Check sheet for the modelled part. Datum: model origin and axes. Units: mm. Coordinates: 2 decimals unless noted, no trailing zeros. Order: outer loops, then holes, each group sorted by start corner. A loop starts at its lowest first (then second) coordinate and runs counter-clockwise, first axis right, second up.
from build123d import *

# Parameters (mm, degrees)
SKETCH1_R           = 86.25
BOSS_EXTRUDE1_DEPTH = 6
SKETCH2_R           = 1.5
CUT_EXTRUDE1_DEPTH  = 6
SKETCH3_R           = 2.25
CUT_EXTRUDE2_DEPTH  = 6
CUT_EXTRUDE3_DEPTH  = 6
FILLET1_R           = 20


with BuildPart() as part:
    # Sketch1 → Boss-Extrude1 (new body)
    with BuildSketch(Plane(origin=(0, 0, 0), x_dir=(1, 0, 0), z_dir=(0, 1, 0))):
        with BuildLine():
            Line((75.993420768, 65), (110, 65))
            Line((110, 65), (110, -65))
            Line((110, -65), (75.993420768, -65))
            ThreePointArc((75.993420768, -65), (0, -100), (-75.993420768, -65))
            Line((-75.993420768, -65), (-110, -65))
            Line((-110, -65), (-110, 65))
            Line((-110, 65), (-75.993420768, 65))
            ThreePointArc((-75.993420768, 65), (0, 100), (75.993420768, 65))
        make_face()
        Circle(SKETCH1_R, mode=Mode.SUBTRACT)
    extrude(amount=BOSS_EXTRUDE1_DEPTH)

    # Sketch2 → Cut-Extrude1 (cut)
    with BuildSketch(Plane(origin=(0, 0, 0), x_dir=(1, 0, 0), z_dir=(0, 1, 0))):
        with Locations((-95.5, 43.5)):
            Circle(SKETCH2_R)
        with Locations((95.5, 43.5)):
            Circle(SKETCH2_R)
        with Locations((95.5, -43.5)):
            Circle(SKETCH2_R)
        with Locations((-95.5, -43.5)):
            Circle(SKETCH2_R)
    extrude(amount=CUT_EXTRUDE1_DEPTH, mode=Mode.SUBTRACT)

    # Sketch3 → Cut-Extrude2 (cut)
    with BuildSketch(Plane(origin=(0, 0, 0), x_dir=(1, 0, 0), z_dir=(0, 1, 0))):
        with Locations((0, 93.125)):
            Circle(SKETCH3_R)
        with Locations((93.125, 0)):
            Circle(SKETCH3_R)
        with Locations((0, -93.125)):
            Circle(SKETCH3_R)
        with Locations((-93.125, 0)):
            Circle(SKETCH3_R)
    extrude(amount=CUT_EXTRUDE2_DEPTH, mode=Mode.SUBTRACT)

    # Sketch4 → Cut-Extrude3 (cut)
    with BuildSketch(Plane(origin=(0, 0, 0), x_dir=(1, 0, 0), z_dir=(0, 1, 0))):
        with BuildLine():
            Line((98.608905775, -36.674701114), (93.856581268, -34.510029742))
            ThreePointArc((93.856581268, -34.510029742), (100, 0), (93.856581268, 34.510029742))
            Line((93.856581268, 34.510029742), (98.608905775, 36.674701114))
            ThreePointArc((98.608905775, 36.674701114), (102.325298886, 46.608905775), (92.391094225, 50.325298886))
            Line((92.391094225, 50.325298886), (87.638769717, 48.160627513))
            ThreePointArc((87.638769717, 48.160627513), (82.248188777, 56.879130117), (75.993420768, 65))
            Line((75.993420768, 65), (110, 65))
            Line((110, 65), (110, -65))
            Line((110, -65), (75.993420768, -65))
            ThreePointArc((75.993420768, -65), (82.248188777, -56.879130117), (87.638769717, -48.160627513))
            Line((87.638769717, -48.160627513), (92.391094225, -50.325298886))
            ThreePointArc((92.391094225, -50.325298886), (102.325298886, -46.608905775), (98.608905775, -36.674701114))
        make_face()
        with BuildLine():
            Line((-98.608905775, 36.674701114), (-93.856581268, 34.510029742))
            ThreePointArc((-93.856581268, 34.510029742), (-100, 0), (-93.856581268, -34.510029742))
            Line((-93.856581268, -34.510029742), (-98.608905775, -36.674701114))
            ThreePointArc((-98.608905775, -36.674701114), (-102.325298886, -46.608905775), (-92.391094225, -50.325298886))
            Line((-92.391094225, -50.325298886), (-87.638769717, -48.160627513))
            ThreePointArc((-87.638769717, -48.160627513), (-82.248188777, -56.879130117), (-75.993420768, -65))
            Line((-75.993420768, -65), (-110, -65))
            Line((-110, -65), (-110, 65))
            Line((-110, 65), (-75.993420768, 65))
            ThreePointArc((-75.993420768, 65), (-82.248188777, 56.879130117), (-87.638769717, 48.160627513))
            Line((-87.638769717, 48.160627513), (-92.391094225, 50.325298886))
            ThreePointArc((-92.391094225, 50.325298886), (-102.325298886, 46.608905775), (-98.608905775, 36.674701114))
        make_face()
    extrude(amount=CUT_EXTRUDE3_DEPTH, mode=Mode.SUBTRACT)

    # Fillet1
    fillet1_edges = [part.edges().sort_by_distance(p)[0] for p in [
        (87.638769717, 3, -48.160627513),
        (93.856581268, 3, -34.510029742),
        (93.856581268, 3, 34.510029742),
        (87.638769717, 3, 48.160627513),
        (-87.638769717, 3, 48.160627513),
        (-93.856581268, 3, 34.510029742),
        (-93.856581268, 3, -34.510029742),
        (-87.638769717, 3, -48.160627513),
    ]]
    fillet(fillet1_edges, radius=FILLET1_R)


solid = part.part
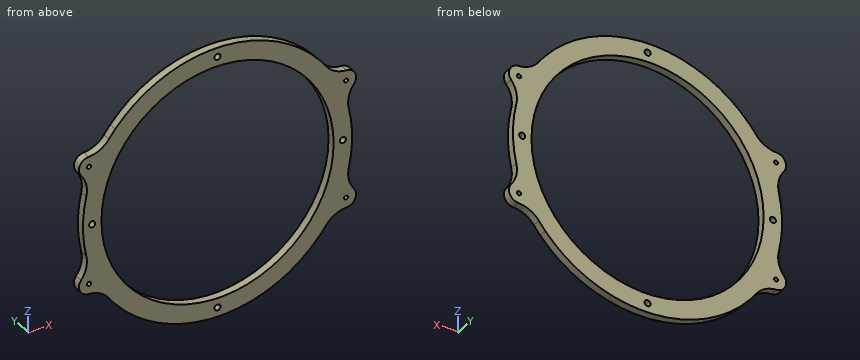
(1) Cross-section at B-B (x = -39). Enter the section's corners in (y, z).
Filled in:
outline: (0, -92.08) - (6, -92.08) - (6, -76.93) - (0, -76.93) - close; (0, 76.93) - (6, 76.93) - (6, 92.08) - (0, 92.08) - close
(2) Cross-section at C-C (y = 4). Count the separate pieces of the cut face and the enclosed holes in it, and give its area (3 significant figures).
Filled in:
separate pieces: 1
enclosed holes: 9
area: 8,830 mm2
(3) Go/stop test with flat-tipped pins: P1, Ø3, axis at y = 3.5, z = 13.5, coming from the +X side; P2, Ø1.5, axis at x = 9.5, y = 5, coming from the +Z side; P3, Ø1.5, axis at y = 0.5, z = -25.5, coming from the -X side. Record where each tip stops, or that it passes through.
Filled in:
P1: stops at x = 99.28
P2: stops at z = 99.62
P3: stops at x = -97.12
(4) Thickness scan on probe 1 along Z at (x, y) = (-95.5, 2.85); probe 2 along X at (y, z) = (2.9, 0) (3 decimals); probe 3 along X at (y, z) = (3, -43.5). Record the ranges inside material, lowest first.
Filled in:
probe 1: z = -51.01 to -45, -42 to 42, 45 to 51.01
probe 2: x = -100 to -95.375, -90.875 to -86.25, 86.25 to 90.875, 95.375 to 100
probe 3: x = -103 to -97, -94 to -74.48, 74.48 to 94, 97 to 103
(5) Cross-section at A-A (x = 57). Enter the section's corners in (y, z), and give its area (3 significant figures).
Filled in:
outline: (0, -82.16) - (6, -82.16) - (6, -64.73) - (0, -64.73) - close; (0, 64.73) - (6, 64.73) - (6, 82.16) - (0, 82.16) - close
area: 209 mm2
